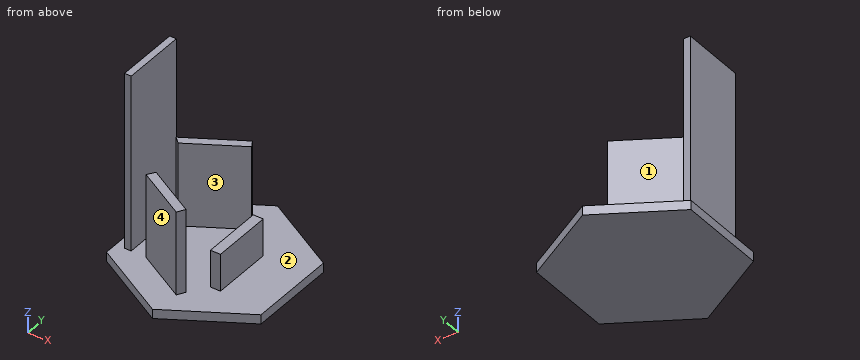
```python
from build123d import *

# Parameters (mm, degrees)
F1_DEPTH = 100
F2_DEPTH = 5
F3_DEPTH = 50
F4_DEPTH = 25


with BuildPart() as f1:
    # F0 (on Top) → F1 (new body)
    with BuildSketch(Plane.XY):
        Polygon((-33.36327, 17.523126), (-37.003014, 17.552711), (-36.847473, -17.309527), (-33.207933, -17.293289), align=None)
    extrude(amount=F1_DEPTH)

    # F0 (on Top) → F2 (join)
    with BuildSketch(Plane.XY):
        Polygon((0.215048, -48.199569), (41.849575, -23.913548), (41.634527, 24.286021), (-0.215048, 48.199569), (-41.849575, 23.913548), (-41.634527, -24.286021), align=None)
        Polygon((2.437659, -33.173904), (-25.006169, -17.492041), (-22.380813, -13.510428), (4.799019, -29.041439), align=None, mode=Mode.SUBTRACT)
        Polygon((11.207818, 13.482378), (16.628671, 13.482378), (16.775963, -19.530714), (11.355217, -19.5549), align=None, mode=Mode.SUBTRACT)
        Polygon((-36.847473, -17.309527), (-37.003014, 17.552711), (-33.36327, 17.523126), (-33.207933, -17.293289), align=None, mode=Mode.SUBTRACT)
        Polygon((-27.306872, 10.376645), (-30.674437, 13.482378), (-1.310807, 30.610607), (0.895825, 26.827686), align=None, mode=Mode.SUBTRACT)
    extrude(amount=F2_DEPTH)

    # F0 (on Top) → F3 (join)
    with BuildSketch(Plane.XY):
        Polygon((-1.310807, 30.610607), (-30.674437, 13.482378), (-27.306872, 10.376645), (0.895825, 26.827686), align=None)
        Polygon((-22.380813, -13.510428), (-25.006169, -17.492041), (2.437659, -33.173904), (4.799019, -29.041439), align=None)
    extrude(amount=F3_DEPTH)

    # F0 (on Top) → F4 (join)
    with BuildSketch(Plane.XY):
        Polygon((16.775963, -19.530714), (16.628671, 13.482378), (11.207818, 13.482378), (11.355217, -19.5549), align=None)
    extrude(amount=F4_DEPTH)


solid = f1.part
```
Geometry: final body of the model. Coordinates: model frame, mm. Face numbers are marked on the shaded views. Coordinates: 2 decimals unless noted, no trailing zeros. Order: outer loops, then holes, each group sorted by start corner. A loop starts at its lowest first (then second) coordinate and runs counter-clockwise, first axis right, second up. Notation, with made-up numbers: (41, 18.5) - (54, 18.5) arc R10 ccw to (54, 29.5) - close; hole circle Ø9 at (-16.5, 68). An arc over 180 degrees is marked (long way). Write each question's results on one line, items separated by ' | '.
(1) Section query D-D, the plane x = -20. Return the cut outline in (y, z).
Values found:
outline: (-36.65, 0) - (36.66, 0) - (36.66, 5) - (19.71, 5) - (19.71, 50) - (14.64, 50) - (14.64, 5) - (-14.87, 5) - (-14.87, 50) - (-20.35, 50) - (-20.35, 5) - (-36.65, 5) - close
(2) First-contact query: pin 1 Ø1.5 at (x, z) = (-22.5, 43.5) entering from -Y; pin 2 Ø10 at (x, z) = (-25, 88) entering from -Y; pin 3 Ø22.5 at (x, y) = (-8, 24) entering from +Z; pin 4 Ø6 at (x, y) = (22, -32.5) entering from +Z. Flat tips, straight axial feed; report the tip coordinate or a pass-through.
Values found:
pin 1: stops at y = -19.35 | pin 2: passes through | pin 3: stops at z = 50 | pin 4: stops at z = 5
(3) Section query B-B, the plane z = 17. Return the cut outline in (x, y), plus the area to 3 significant figures.
Values found:
outline: (-37, 17.55) - (-36.85, -17.31) - (-33.21, -17.29) - (-33.36, 17.52) - close; (-30.67, 13.48) - (-27.31, 10.38) - (0.9, 26.83) - (-1.31, 30.61) - close; (-25.01, -17.49) - (2.44, -33.17) - (4.8, -29.04) - (-22.38, -13.51) - close; (11.21, 13.48) - (11.36, -19.55) - (16.78, -19.53) - (16.63, 13.48) - close | area: 601 mm²
(4) Section query C-C, the plane y = 5.5. Return the cut outline in (x, z).
Values found:
outline: (-41.77, 0) - (41.72, 0) - (41.72, 5) - (16.66, 5) - (16.66, 25) - (11.24, 25) - (11.24, 5) - (-33.31, 5) - (-33.31, 100) - (-36.95, 100) - (-36.95, 5) - (-41.77, 5) - close
(5) Mould query, pull axis Y, two halves, no side actions, for the marked faces 1, 2, 3 and 4. Classes: +Y half, -Y half, draft (parallel to the pull), parting line (faces both ways), or undercut.
Values found:
face 1: +Y half | face 2: undercut | face 3: undercut | face 4: -Y half
(6) Section query A-A, the plane z = 42.5. Return the cut outline in (x, y).
Values found:
outline: (-37, 17.55) - (-36.85, -17.31) - (-33.21, -17.29) - (-33.36, 17.52) - close; (-30.67, 13.48) - (-27.31, 10.38) - (0.9, 26.83) - (-1.31, 30.61) - close; (-25.01, -17.49) - (2.44, -33.17) - (4.8, -29.04) - (-22.38, -13.51) - close
(7) Line query: line 1 (Z direction, x = -7, y = -31); line 2 (X direction, y = 3, z = 11.5); line 3 (Y direction, x = -24, z = 24.5). Output: solid intervals per line, ascending. Write a range as [from, to].
Values found:
line 1: z = [0, 5] | line 2: x = [-36.94, -33.3], [11.25, 16.68] | line 3: y = [-18.07, -15.97], [12.31, 17.38]
